Could you check a few things on this model? Use its own coordinates, in mm. Face numbers are marked on the shaded views. A direction names the side the tool comes from. Coordinates: 2 decimals unless noted, no trailing zeros. Order: outer loops, then holes, each group sorted by start corner. A loop starts at its lowest first (then second) coordinate and runs counter-clockwise, first axis right, second up. Notation, with made-up numbers: (18, 18.25) - (57, 18.25) arc R25 cw to (57, 42.25) - close; hole circle Ø7 at (21, 71.5). An arc over 180 degrees is marked (long way). One line per item, written item: value.
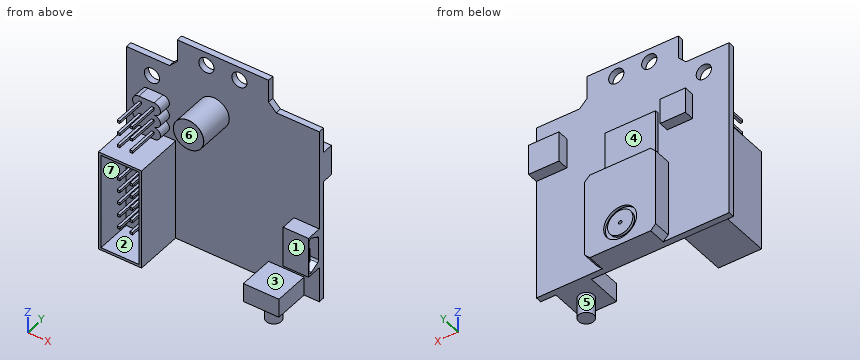
from build123d import *

# Parameters (mm, degrees)
SKETCH_1_R          = 1.5
EXTRUDE_1_DEPTH     = 1.2
EXTRUDE_2_DEPTH     = 3.5
SKETCH_3_R          = 3.25
SKETCH_3_R_2        = 2.5
CUT_EXTRUDE_1_DEPTH = 0.5
SKETCH_4_R          = 0.35
CUT_EXTRUDE_2_DEPTH = 0.7
SKETCH_5_W          = 6
SKETCH_5_H          = 6
EXTRUDE_3_DEPTH     = 2.2
SKETCH_6_W          = 10
SKETCH_6_H          = 10
EXTRUDE_4_DEPTH     = 0.7
SKETCH_7_W          = 5
SKETCH_7_H          = 5
EXTRUDE_5_DEPTH     = 2
SKETCH_8_W          = 5
SKETCH_8_H          = 8
EXTRUDE_6_DEPTH     = 3
CUT_EXTRUDE_3_DEPTH = 2.5
SKETCH_10_W         = 2.8
SKETCH_10_H         = 0.3
EXTRUDE_7_DEPTH     = 2.3
SKETCH_11_R         = 3
EXTRUDE_8_DEPTH     = 7.1
FILLET_1_R          = 0.02
SKETCH_12_W         = 7
SKETCH_12_H         = 3.7
EXTRUDE_9_DEPTH     = 7
SKETCH_13_R         = 1.5
EXTRUDE_10_DEPTH    = 4.1
SKETCH_14_W         = 8.5
SKETCH_14_H         = 20
SKETCH_14_W_2       = 7.5
SKETCH_14_H_2       = 19
EXTRUDE_11_DEPTH    = 9.5
SKETCH_15_W         = 0.5
SKETCH_15_H         = 0.5
EXTRUDE_12_DEPTH    = 8.5
SKETCH_16_W         = 0.5
SKETCH_16_H         = 0.5
EXTRUDE_13_DEPTH    = 8.5
SKETCH_17_W         = 7.5
SKETCH_17_H         = 19
EXTRUDE_14_DEPTH    = 2.5


with BuildPart() as part:
    # Sketch 1 → Extrude 1 (new body)
    with BuildSketch(Plane(origin=(0, 0, 0), x_dir=(1, 0, 0), z_dir=(0, 1, 0))):
        Polygon((10.5, -17.5), (19, -17.5), (19, 17.5), (-19, 17.5), (-19, -17.5), (-10.5, -17.5), (-9, -19), (-9, -23.5), (9, -23.5), (9, -19), align=None)
        with Locations(Location((-3.25, -20.9, 0), (0, 0, 270))):
            Circle(SKETCH_1_R, mode=Mode.SUBTRACT)
        with Locations(Location((3.25, -20.9, 0), (0, 0, 270))):
            Circle(SKETCH_1_R, mode=Mode.SUBTRACT)
        with Locations(Location((-14, -13.8, 0), (0, 0, 270))):
            Circle(SKETCH_1_R, mode=Mode.SUBTRACT)
    extrude(amount=-EXTRUDE_1_DEPTH)

    # Sketch 2 → Extrude 2 (add)
    with BuildSketch(Plane(origin=(0, 0, 0), x_dir=(1, 0, 0), z_dir=(0, 1, 0))):
        Polygon((-6, 17.5), (6, 17.5), (7, 16.5), (7, 1.5), (6, 0.5), (-6, 0.5), (-7, 1.5), (-7, 16.5), align=None)
    extrude(amount=EXTRUDE_2_DEPTH)

    # Sketch 3 → Cut-Extrude 1 (cut)
    with BuildSketch(Plane(origin=(0, 3.5, 0), x_dir=(1, 0, 0), z_dir=(0, 1, 0))):
        with Locations(Location((0, 13, 0), (0, 0, 270))):
            Circle(SKETCH_3_R)
        with Locations(Location((0, 13, 0), (0, 0, 270))):
            Circle(SKETCH_3_R_2, mode=Mode.SUBTRACT)
    extrude(amount=-CUT_EXTRUDE_1_DEPTH, mode=Mode.SUBTRACT)

    # Sketch 4 → Cut-Extrude 2 (cut)
    with BuildSketch(Plane(origin=(0, 3.5, 0), x_dir=(1, 0, 0), z_dir=(0, 1, 0))):
        with Locations(Location((0, 13, 0), (0, 0, 270))):
            Circle(SKETCH_4_R)
    extrude(amount=-CUT_EXTRUDE_2_DEPTH, mode=Mode.SUBTRACT)

    # Sketch 5 → Extrude 3 (add)
    with BuildSketch(Plane(origin=(0, 0, 0), x_dir=(1, 0, 0), z_dir=(0, 1, 0))):
        with Locations((16, -9.5)):
            Rectangle(SKETCH_5_W, SKETCH_5_H)
    extrude(amount=EXTRUDE_3_DEPTH)

    # Sketch 6 → Extrude 4 (add)
    with BuildSketch(Plane(origin=(0, 0, 0), x_dir=(1, 0, 0), z_dir=(0, 1, 0))):
        with Locations((0, -4.5)):
            Rectangle(SKETCH_6_W, SKETCH_6_H)
    extrude(amount=EXTRUDE_4_DEPTH)

    # Sketch 7 → Extrude 5 (add)
    with BuildSketch(Plane(origin=(0, 0, 0), x_dir=(1, 0, 0), z_dir=(0, 1, 0))):
        with Locations((-9.3, -7.7)):
            Rectangle(SKETCH_7_W, SKETCH_7_H)
    extrude(amount=EXTRUDE_5_DEPTH)

    # Sketch 8 → Extrude 6 (add)
    with BuildSketch(Plane.XZ.offset(1.2)):
        with Locations((16.5, -6.5)):
            Rectangle(SKETCH_8_W, SKETCH_8_H)
    extrude(amount=EXTRUDE_6_DEPTH)

    # Sketch 9 → Cut-Extrude 3 (cut)
    with BuildSketch(Plane(origin=(19, 0, 0), x_dir=(0, 0, -1), z_dir=(1, 0, 0))):
        with BuildLine():
            Line((3.860082228, -1.669841418), (2.978600746, -3.369841418))
            ThreePointArc((2.978600746, -3.369841418), (2.995231426, -3.859731312), (3.422478012, -4.1))
            Line((3.422478012, -4.1), (9.577521988, -4.1))
            ThreePointArc((9.577521988, -4.1), (10.004768574, -3.859731312), (10.021399254, -3.369841418))
            Line((10.021399254, -3.369841418), (9.139917772, -1.669841418))
            ThreePointArc((9.139917772, -1.669841418), (8.955771818, -1.472753414), (8.696040506, -1.4))
            Line((8.696040506, -1.4), (4.303959494, -1.4))
            ThreePointArc((4.303959494, -1.4), (4.044228182, -1.472753414), (3.860082228, -1.669841418))
        make_face()
    extrude(amount=-CUT_EXTRUDE_3_DEPTH, mode=Mode.SUBTRACT)

    # Sketch 10 → Extrude 7 (add)
    with BuildSketch(Plane(origin=(16.5, 0, 0), x_dir=(0, 0, -1), z_dir=(1, 0, 0))):
        with Locations((6.5, -3.65)):
            Rectangle(SKETCH_10_W, SKETCH_10_H)
    extrude(amount=EXTRUDE_7_DEPTH)

    # Sketch 11 → Extrude 8 (add)
    with BuildSketch(Plane(origin=(0, -1.2, 0), x_dir=(-1, 0, 0), z_dir=(0, -1, 0))):
        with Locations(Location((1.75, -11.9, 0), (0, 0, 270))):
            Circle(SKETCH_11_R)
    extrude(amount=EXTRUDE_8_DEPTH)

    # Fillet 1
    fillet_1_edges = [part.edges().sort_by_distance(p)[0] for p in [
        (-1.75, -8.3, 8.9),
    ]]
    fillet(fillet_1_edges, radius=FILLET_1_R)

    # Sketch 12 → Extrude 9 (add)
    with BuildSketch(Plane.XZ.offset(1.2)):
        with Locations((12.5, -15.65)):
            Rectangle(SKETCH_12_W, SKETCH_12_H)
    extrude(amount=EXTRUDE_9_DEPTH)

    # Sketch 13 → Extrude 10 (add)
    with BuildSketch(Plane(origin=(0, 0, -17.5), x_dir=(-1, 0, 0), z_dir=(0, 0, -1))):
        with Locations(Location((-12.5, -4.7, 0), (0, 0, 180))):
            Circle(SKETCH_13_R)
    extrude(amount=EXTRUDE_10_DEPTH)

    # Sketch 14 → Extrude 11 (add)
    with BuildSketch(Plane.XZ.offset(1.2)):
        with Locations((-13.55, -7.45)):
            Rectangle(SKETCH_14_W, SKETCH_14_H)
        with Locations((-13.55, -7.45)):
            Rectangle(SKETCH_14_W_2, SKETCH_14_H_2, mode=Mode.SUBTRACT)
    extrude(amount=EXTRUDE_11_DEPTH)

    # Sketch 15 → Extrude 12 (add)
    with BuildSketch(Plane.XZ.offset(1.2)):
        with Locations((-14.55, -2.2)):
            Rectangle(SKETCH_15_W, SKETCH_15_H)
        with Locations((-12.05, -2.2)):
            Rectangle(SKETCH_15_W, SKETCH_15_H)
        with Locations((-12.05, -4.7)):
            Rectangle(SKETCH_15_W, SKETCH_15_H)
        with Locations((-12.05, -7.2)):
            Rectangle(SKETCH_15_W, SKETCH_15_H)
        with Locations((-12.05, -9.7)):
            Rectangle(SKETCH_15_W, SKETCH_15_H)
        with Locations((-12.05, -12.2)):
            Rectangle(SKETCH_15_W, SKETCH_15_H)
        with Locations((-14.55, -4.7)):
            Rectangle(SKETCH_15_W, SKETCH_15_H)
        with Locations((-14.55, -7.2)):
            Rectangle(SKETCH_15_W, SKETCH_15_H)
        with Locations((-14.55, -9.7)):
            Rectangle(SKETCH_15_W, SKETCH_15_H)
        with Locations((-14.55, -12.2)):
            Rectangle(SKETCH_15_W, SKETCH_15_H)
    extrude(amount=EXTRUDE_12_DEPTH)

    # Sketch 16 → Extrude 13 (add)
    with BuildSketch(Plane.XZ.offset(1.2)):
        with Locations((-14.55, 4.6)):
            Rectangle(SKETCH_16_W, SKETCH_16_H)
        with Locations((-12.05, 4.6)):
            Rectangle(SKETCH_16_W, SKETCH_16_H)
        with Locations((-12.05, 7.1)):
            Rectangle(SKETCH_16_W, SKETCH_16_H)
        with Locations((-12.05, 9.6)):
            Rectangle(SKETCH_16_W, SKETCH_16_H)
        with Locations((-14.55, 7.1)):
            Rectangle(SKETCH_16_W, SKETCH_16_H)
        with Locations((-14.55, 9.6)):
            Rectangle(SKETCH_16_W, SKETCH_16_H)
    extrude(amount=EXTRUDE_13_DEPTH)

    # Sketch 17 → Extrude 14 (add)
    with BuildSketch(Plane.XZ.offset(1.2)):
        with Locations((-13.55, -7.45)):
            Rectangle(SKETCH_17_W, SKETCH_17_H)
        with BuildLine():
            Line((-14.8, 10.85), (-11.8, 10.85))
            ThreePointArc((-11.8, 10.85), (-10.55, 9.6), (-11.8, 8.35))
            ThreePointArc((-11.8, 8.35), (-10.55, 7.1), (-11.8, 5.85))
            ThreePointArc((-11.8, 5.85), (-10.55, 4.6), (-11.8, 3.35))
            Line((-11.8, 3.35), (-14.8, 3.35))
            ThreePointArc((-14.8, 3.35), (-16.05, 4.6), (-14.8, 5.85))
            ThreePointArc((-14.8, 5.85), (-16.05, 7.1), (-14.8, 8.35))
            ThreePointArc((-14.8, 8.35), (-16.05, 9.6), (-14.8, 10.85))
        make_face()
    extrude(amount=EXTRUDE_14_DEPTH)


solid = part.part
Item 1: I'm going to push flat-ended pins straight in: pin 1 Ø1.5 at (x, y) = (-14.5, -1.5) entering from +Z; pin 2 Ø0.6 at (y, z) = (-6.5, -9.5) entering from -X; pin 3 Ø3 at (y, z) = (-7.5, 4.5) entering from +X. Where does each tip first touch, or does it pass through?
Conclusion:
pin 1: z = 17.5
pin 2: x = -17.8
pin 3: x = -11.8
Item 2: I want a section at D-D on x = 11.5. Please give me the cut outline in (y, z).
Conclusion:
outline: (-8.2, -17.5) - (-5.82, -17.5) - (-5.82, -21.6) - (-3.58, -21.6) - (-3.58, -17.5) - (0, -17.5) - (0, 17.5) - (-1.2, 17.5) - (-1.2, -13.8) - (-8.2, -13.8) - close
Item 3: For the marked faces 1, 2, 3 and 4, which set-ups out of +Z, -Z, +X, -X, +Y, -Y let a thin tool reach every point of the face, with its end or its side?
Conclusion:
face 1: +Z, +X, -Y
face 2: -Y
face 3: +X, -Y
face 4: +Z, +Y
Item 4: If I drill on probe 1 along X at (y, z) = (3.1, -13); probe 2 along X at (y, z) = (-4.75, -16); probe 3 along X at (y, z) = (-0.5, 20.9), over which ranges is the centre line in solid material (lowest first)?
Conclusion:
probe 1: -7 to -3.25, -2.5 to -0.35, 0.35 to 2.5, 3.25 to 7
probe 2: -17.8 to -17.3, -9.8 to -9.3, 9 to 16
probe 3: -9 to -4.75, -1.75 to 1.75, 4.75 to 9
Item 5: I want a section at C-C on z = 16. Please give me the cut outline in (x, y).
Conclusion:
outline: (-19, -1.2) - (19, -1.2) - (19, 0) - (-19, 0) - close
Item 6: I want a section at A-A on x = -13. Please give me the cut outline in (y, z), then the cut area to 3 significant figures.
Conclusion:
outline: (-10.7, -17.45) - (-1.2, -17.45) - (-1.2, -17.5) - (0, -17.5) - (0, 12.68) - (-1.2, 12.68) - (-1.2, 10.85) - (-3.7, 10.85) - (-3.7, 3.35) - (-1.2, 3.35) - (-1.2, 2.55) - (-10.7, 2.55) - (-10.7, 2.05) - (-3.7, 2.05) - (-3.7, -16.95) - (-10.7, -16.95) - close; (-1.2, 14.92) - (0, 14.92) - (0, 17.5) - (-1.2, 17.5) - close
area: 115 mm²
Item 7: I want a section at B-B on y = -5.25. Give the number of separate pieces and of enclosed holes in the cut face, then the cut area to 3 significant figures.
Conclusion:
separate pieces: 19
enclosed holes: 1
area: 97.1 mm²
Item 8: Thinking about a two-plate mould opening in X: for the marked faces 5, 6 and 7, which applies, pulls with the +X half, pulls with the -X half, needs draft (parallel to the pull), parting line crosses it, or undercut?
Conclusion:
face 5: parting line crosses it
face 6: needs draft
face 7: undercut
